from build123d import *

# Parameters (mm, degrees)
F2_R     = 1
F3_W     = 1.2023348827
F3_H     = 4.3877884746
F4_DEPTH = 7
F5_W     = 1.6818879384
F5_H     = 3
F5_W_2   = 1.39512593
F6_DEPTH = 12.5


with BuildPart() as f1:
    # F0 (on Front) → F1 (revolve)
    with BuildSketch(Plane.XZ):
        Polygon((5.5, 4.8), (2, 4.8), (2, 0.0084556759), (0, 0.0084556759), (0, -12.2), (5, -12.2), (5, -3), (4, -3), (4, 0), (5.5, 0), align=None)
    revolve(axis=Axis((0, 0, 13.3898657501), (0, 0, -1)))

    # F2
    f2_edges = [f1.edges().sort_by_distance(p)[0] for p in [
        (-5.5, 0, 4.8),
        (-2, 0, 4.8),
    ]]
    fillet(f2_edges, radius=F2_R)

    # F3 (on face) → F4 (join)
    with BuildSketch(Plane(origin=(0, 0, -12.2), x_dir=(1, 0, 0), z_dir=(0, 0, -1))):
        Rectangle(F3_W, F3_H)
    extrude(amount=F4_DEPTH)

    # F5 (on Right) → F6 (cut, symmetric)
    with BuildSketch(Plane.YZ):
        with Locations((3.8409439692, -1.5)):
            Rectangle(F5_W, F5_H)
        with Locations((-3.697562965, -1.5)):
            Rectangle(F5_W_2, F5_H)
    extrude(amount=F6_DEPTH, both=True, mode=Mode.SUBTRACT)


solid = f1.part
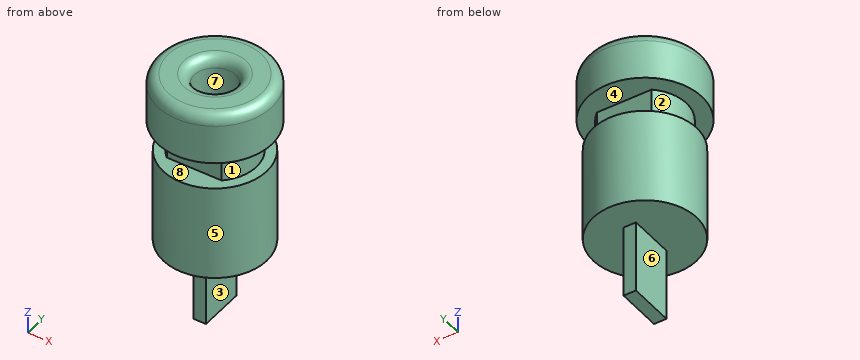
Design review of the part built by this model. Coordinates are the model's own, in mm. Face numbers are marked on the shaded views. A direction names the side the tool comes from. Coordinates: 2 decimals unless noted, no trailing zeros. Order: outer loops, then holes, each group sorted by start corner. A loop starts at its lowest first (then second) coordinate and runs counter-clockwise, first axis right, second up. Notation, with made-up numbers: (-13.5, 22.25) -> (-4.5, 22.25) arc R30 ccw to (-4.5, 54.25) -> close; hole circle Ø11 at (-3, 44.5). An arc over 180 degrees is marked (long way). Use one line per item in the form item = value. Start each with the question number.
(1) Insertion check: pin 1 (5 mm diameter, centred on y = -0.5, z = -14.5, fed in from -X); pin 2 (1 mm diameter, centred on y = 3, z = -10.5, fed in from +X); pin 3 (1 mm diameter, centred on x = 0, y = 3, fed in from -Z). Each pin has a flat end and moves straight along its axis. Give the tip position at first contact, or say it passes through.
(2) Add section A-A on x = 0. State the section outline as (y, z) points, plus the area to 3 significant figures.
(3) The part is to be moulded in two halves that separate along X. For the marked faces 6, 7 and 8, say which applies: +X half, -X half, draft (parallel to the pull), parting line (faces both ways), or undercut.
(4) For probe 1 along X at (y, z) = (0, 1.9); probe 2 along Z at (x, y) = (0.25, -4.5), list the stretches that pass through material, from the lowest coordinate up.
(5) For the marked faces 1, 2, 3, 4 and 5, list the 3-axis set-ups (+Z, -Z, +X, -X, +Y, -Y) from which the entire face can be reached by the end or side of a thin tool; tool diameter is ignored.
(6) Add section D-D on z = -2. State the section outline as (x, y) points, plus the area to 3 significant figures.
(7) Add section B-B on y = 0. State the section outline as (x, z) points.
(8) Add section C-C on z = 2.75. State the section outline as (x, y) points, plus the area to 3 significant figures.
Answer block:
q1.pin_1 = -5
q1.pin_2 = 4.33
q1.pin_3 = -12.2
q2.outline = (-5.5, 0) -> (-3, 0) -> (-3, -3) -> (-5, -3) -> (-5, -12.2) -> (-2.19, -12.2) -> (-2.19, -19.2) -> (2.19, -19.2) -> (2.19, -12.2) -> (5, -12.2) -> (5, -3) -> (3, -3) -> (3, 0) -> (5.5, 0) -> (5.5, 3.8) arc R1 ccw to (4.5, 4.8) -> (3, 4.8) arc R1 ccw to (2, 3.8) -> (2, 0.01) -> (-2, 0.01) -> (-2, 3.8) arc R1 ccw to (-3, 4.8) -> (-4.5, 4.8) arc R1 ccw to (-5.5, 3.8) -> close
q2.area = 173 mm²
q3.face_6 = -X half
q3.face_7 = undercut
q3.face_8 = draft
q4.probe_1 = -5.5 to -2, 2 to 5.5
q4.probe_2 = -12.2 to -3, 0 to 4.8
q5.face_1 = +X
q5.face_2 = -X
q5.face_3 = -Z, +X, +Y, -Y
q5.face_4 = none
q5.face_5 = -Z
q6.outline = (-2.65, -3) -> (2.65, -3) arc R4 ccw to (2.65, 3) -> (-2.65, 3) arc R4 ccw to start
q6.area = 43.0 mm²
q7.outline = (-5.5, 0) -> (-4, 0) -> (-4, -3) -> (-5, -3) -> (-5, -12.2) -> (-0.6, -12.2) -> (-0.6, -19.2) -> (0.6, -19.2) -> (0.6, -12.2) -> (5, -12.2) -> (5, -3) -> (4, -3) -> (4, 0) -> (5.5, 0) -> (5.5, 3.8) arc R1 ccw to (4.5, 4.8) -> (3, 4.8) arc R1 ccw to (2, 3.8) -> (2, 0.01) -> (-2, 0.01) -> (-2, 3.8) arc R1 ccw to (-3, 4.8) -> (-4.5, 4.8) arc R1 ccw to (-5.5, 3.8) -> close
q8.outline = circle Ø11 at (0, 0); hole circle Ø4 at (0, 0)
q8.area = 82.5 mm²
